```python
from build123d import *

# Parameters (mm, degrees)
ENL_V_MAT_EXTRU_1_DEPTH = 20.395702365


with BuildPart() as part:
    # Esquisse1 → Révolution1 (revolve)
    with BuildSketch(Plane.XY, mode=Mode.PRIVATE) as r_volution1_sk:
        Polygon((157.568040745, 0), (157.568040745, 5), (158.36383893, 5), (158.36383893, 10), (159.159637116, 10), (159.159637116, 15), (170, 15), (170, 20), (137.568040745, 20), (137.568040745, 0), align=None)
    revolve(r_volution1_sk.sketch.rotate(Axis((0, 0, 0), (0, 1, 0)), 90), axis=Axis((0, 0, 0), (0, 1, 0)))

    # Esquisse2 → Enlèv. mat.-Extru.1 (cut)
    with BuildSketch(Plane.XZ.offset(-15)):
        Polygon((-9.406937207, -131.726748145), (-11.551478732, -172.647038111), (-6.558331058, -172.908717892), (-4.413789534, -131.988427927), align=None)
    extrude(amount=ENL_V_MAT_EXTRU_1_DEPTH, mode=Mode.SUBTRACT)


solid = part.part
```
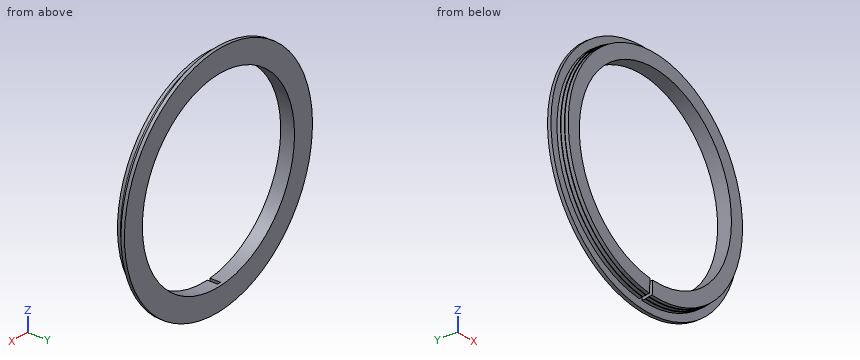
Design review of the part built by this model. Coordinates are the model's own, in mm. Give positions to 0.01 mm unless a question says otherwise; leave off trailing zeros. Order: outer loops, then holes, each group sorted by start corner. A loop starts at its lowest first (then second) coordinate and runs counter-clockwise, first axis right, second up. Notation, with made-up numbers: (0, 37.25) -> (7, 37.25) arc R31 ccw to (7, 61.25) -> close; hole circle Ø2 at (-21, -11.5). An arc over 180 degrees is marked (long way). Write item = value, one per line. Start each with the question number.
(1) We need section B-B on x = 0. Write out the cut boundary in (y, z).
(2) For pin 1 (5 mm diameter, centred on x = -41, y = 16, fed in from -Z); pin 2 (5 mm diameter, centred on y = 5, z = -47.5, fed in from +X); pin 3 (1.5 mm diameter, centred on x = -120, y = 2.5, fed in from -Z), all flat-tipped, find the tip position at first contact; note any pin that passes through.
(3) We need section A-A on z = 0. Write out the cut boundary in (x, y).
(4) To check wall thickness, follow line 1 along X through (y, z) = (8.5, -65.5); line 2 along X through (y, z) = (13.5, 0); line 3 along Z through (x, y) = (5.5, 13.75). State the ranges of each line that lie inside material, in increasing order.
Numbers:
q1.outline = (0, -157.57) -> (5, -157.57) -> (5, -158.36) -> (10, -158.36) -> (10, -159.16) -> (15, -159.16) -> (15, -170) -> (20, -170) -> (20, -137.57) -> (0, -137.57) -> close; (0, 137.57) -> (20, 137.57) -> (20, 170) -> (15, 170) -> (15, 159.16) -> (10, 159.16) -> (10, 158.36) -> (5, 158.36) -> (5, 157.57) -> (0, 157.57) -> close
q2.pin_1 = -165.58
q2.pin_2 = 151.84
q2.pin_3 = -102.99
q3.outline = (-170, 15) -> (-159.16, 15) -> (-159.16, 10) -> (-158.36, 10) -> (-158.36, 5) -> (-157.57, 5) -> (-157.57, 0) -> (-137.57, 0) -> (-137.57, 20) -> (-170, 20) -> close; (137.57, 0) -> (157.57, 0) -> (157.57, 5) -> (158.36, 5) -> (158.36, 10) -> (159.16, 10) -> (159.16, 15) -> (170, 15) -> (170, 20) -> (137.57, 20) -> close
q4.line_1 = -144.18 to -120.97, 120.97 to 144.18
q4.line_2 = -159.16 to -137.57, 137.57 to 159.16
q4.line_3 = -159.06 to -137.46, 137.46 to 159.06
